Model file for the job. Use its own axes, mm. Round coordinates to 2 decimals unless told otherwise and drop trailing zeros. Loops run counter-clockwise (first coordinate to the right, second up) from the corner with the lowest first, then second, coordinate; pieces in that order, holes last. Notation, with made-up numbers: (38.25, 41.5) -> (92.25, 41.5) arc R20 cw to (92.25, 64.5) -> close; hole circle Ø10 at (5, 58). An arc over 180 degrees is marked (long way). Use a Markdown table: item, result.
from build123d import *

# Parameters (mm, degrees)
BOSS_EXTRUDE3_DEPTH = 200
CHAMFER2_SIZE       = 18
CHAMFER3_SIZE       = 18
SKETCH6_W           = 200
SKETCH6_H           = 8
CUT_EXTRUDE2_DEPTH  = 4
SKETCH7_W           = 200
SKETCH7_H           = 8
CUT_EXTRUDE3_DEPTH  = 4
SKETCH8_R           = 1.4
CUT_EXTRUDE4_DEPTH  = 3
SKETCH9_R           = 2.1
CUT_EXTRUDE5_DEPTH  = 6
SKETCH10_R          = 2.1
CUT_EXTRUDE6_DEPTH  = 6
CUT_EXTRUDE7_DEPTH  = 4
SKETCH12_W          = 4
SKETCH12_H          = 10
SKETCH12_W_2        = 10
SKETCH12_H_2        = 4
CUT_EXTRUDE8_DEPTH  = 14
FILLET1_R           = 4
FILLET2_R           = 4
SKETCH13_W          = 4
SKETCH13_H          = 10
SKETCH13_W_2        = 10
SKETCH13_H_2        = 4
CUT_EXTRUDE9_DEPTH  = 14
FILLET3_R           = 4
SKETCH14_R          = 2.1
CUT_EXTRUDE10_DEPTH = 4
SKETCH15_R          = 2.1
CUT_EXTRUDE11_DEPTH = 4
SKETCH16_R          = 2.1
CUT_EXTRUDE12_DEPTH = 4


with BuildPart() as part:
    # Sketch5 → Boss-Extrude3 (new body)
    with BuildSketch(Plane(origin=(0, 0, 0), x_dir=(0, 0, -1), z_dir=(1, 0, 0))):
        Polygon((0, 0), (0, 36), (8, 36), (8, 8), (36, 8), (36, 0), align=None)
    extrude(amount=BOSS_EXTRUDE3_DEPTH)

    # Chamfer2
    chamfer2_edges = [part.edges().sort_by_distance(p)[0] for p in [
        (100, 8, -8),
    ]]
    chamfer(chamfer2_edges, length=CHAMFER2_SIZE)

    # Chamfer3
    chamfer3_edges = [part.edges().sort_by_distance(p)[0] for p in [
        (100, 0, 0),
    ]]
    chamfer(chamfer3_edges, length=CHAMFER3_SIZE)

    # Sketch6 → Cut-Extrude2 (cut)
    with BuildSketch(Plane(origin=(0, 0, 0), x_dir=(-1, 0, 0), z_dir=(0, -1, 0))):
        with Locations((-100, 32)):
            Rectangle(SKETCH6_W, SKETCH6_H)
    extrude(amount=-CUT_EXTRUDE2_DEPTH, mode=Mode.SUBTRACT)

    # Sketch7 → Cut-Extrude3 (cut)
    with BuildSketch(Plane.XY):
        with Locations((100, 32)):
            Rectangle(SKETCH7_W, SKETCH7_H)
    extrude(amount=-CUT_EXTRUDE3_DEPTH, mode=Mode.SUBTRACT)

    # Sketch8 → Cut-Extrude4 (cut)
    with BuildSketch(Plane(origin=(0, 17, -17), x_dir=(-1, 0, 0), z_dir=(0, 0.7071067811865438, -0.7071067811865512))):
        with Locations(Location((-182.5, 0, 0), (0, 0, 90))):
            Circle(SKETCH8_R)
        with Locations(Location((-167.5, 0, 0), (0, 0, 90))):
            Circle(SKETCH8_R)
        with Locations(Location((-152.5, 0, 0), (0, 0, 90))):
            Circle(SKETCH8_R)
        with Locations(Location((-137.5, 0, 0), (0, 0, 90))):
            Circle(SKETCH8_R)
        with Locations(Location((-122.5, 0, 0), (0, 0, 90))):
            Circle(SKETCH8_R)
        with Locations(Location((-107.5, 0, 0), (0, 0, 90))):
            Circle(SKETCH8_R)
        with Locations(Location((-92.5, 0, 0), (0, 0, 90))):
            Circle(SKETCH8_R)
        with Locations(Location((-77.5, 0, 0), (0, 0, 90))):
            Circle(SKETCH8_R)
        with Locations(Location((-62.5, 0, 0), (0, 0, 90))):
            Circle(SKETCH8_R)
        with Locations(Location((-47.5, 0, 0), (0, 0, 90))):
            Circle(SKETCH8_R)
        with Locations(Location((-32.5, 0, 0), (0, 0, 90))):
            Circle(SKETCH8_R)
        with Locations(Location((-17.5, 0, 0), (0, 0, 90))):
            Circle(SKETCH8_R)
    extrude(amount=-CUT_EXTRUDE4_DEPTH, mode=Mode.SUBTRACT)

    # Sketch9 → Cut-Extrude5 (cut)
    with BuildSketch(Plane(origin=(0, 17, -17), x_dir=(-1, 0, 0), z_dir=(0, 0.7071067811865438, -0.7071067811865512))):
        with Locations(Location((-73, -10, 0), (0, 0, 90))):
            Circle(SKETCH9_R)
        with Locations(Location((-127, -10, 0), (0, 0, 90))):
            Circle(SKETCH9_R)
        with Locations(Location((-127, 10, 0), (0, 0, 90))):
            Circle(SKETCH9_R)
        with Locations(Location((-73, 10, 0), (0, 0, 90))):
            Circle(SKETCH9_R)
    extrude(amount=-CUT_EXTRUDE5_DEPTH, mode=Mode.SUBTRACT)

    # Sketch10 → Cut-Extrude6 (cut)
    with BuildSketch(Plane(origin=(0, 17, -17), x_dir=(-1, 0, 0), z_dir=(0, 0.7071067811865438, -0.7071067811865512))):
        with Locations(Location((-89, -10, 0), (0, 0, 90))):
            Circle(SKETCH10_R)
        with Locations(Location((-111, -10, 0), (0, 0, 90))):
            Circle(SKETCH10_R)
        with Locations(Location((-111, 10, 0), (0, 0, 90))):
            Circle(SKETCH10_R)
        with Locations(Location((-89, 10, 0), (0, 0, 90))):
            Circle(SKETCH10_R)
    extrude(amount=-CUT_EXTRUDE6_DEPTH, mode=Mode.SUBTRACT)

    # Sketch11 → Cut-Extrude7 (cut)
    with BuildSketch(Plane(origin=(0, 17, -17), x_dir=(-1, 0, 0), z_dir=(0, 0.7071067811865438, -0.7071067811865512))):
        Polygon((0, -12), (-14, 0), (0, 12), align=None)
        Polygon((-200, 12), (-186, 0), (-200, -12), align=None)
    extrude(amount=-CUT_EXTRUDE7_DEPTH, mode=Mode.SUBTRACT)

    # Sketch12 → Cut-Extrude8 (cut)
    with BuildSketch(Plane(origin=(200, 0, 0), x_dir=(0, 0, -1), z_dir=(1, 0, 0))):
        with Locations((2, 23)):
            Rectangle(SKETCH12_W, SKETCH12_H)
        with Locations((23, 2)):
            Rectangle(SKETCH12_W_2, SKETCH12_H_2)
    extrude(amount=-CUT_EXTRUDE8_DEPTH, mode=Mode.SUBTRACT)

    # Fillet1
    fillet1_edges = [part.edges().sort_by_distance(p)[0] for p in [
        (14, 15.585786438, -15.585786438),
        (186, 15.585786438, -15.585786438),
    ]]
    fillet(fillet1_edges, radius=FILLET1_R)

    # Fillet2
    fillet2_edges = [part.edges().sort_by_distance(p)[0] for p in [
        (186, 18, -2),
        (186, 2, -18),
    ]]
    fillet(fillet2_edges, radius=FILLET2_R)

    # Sketch13 → Cut-Extrude9 (cut)
    with BuildSketch(Plane.ZY):
        with Locations((-2, 23)):
            Rectangle(SKETCH13_W, SKETCH13_H)
        with Locations((-23, 2)):
            Rectangle(SKETCH13_W_2, SKETCH13_H_2)
    extrude(amount=-CUT_EXTRUDE9_DEPTH, mode=Mode.SUBTRACT)

    # Fillet3
    fillet3_edges = [part.edges().sort_by_distance(p)[0] for p in [
        (14, 18, -2),
        (14, 2, -18),
    ]]
    fillet(fillet3_edges, radius=FILLET3_R)

    # Sketch14 → Cut-Extrude10 (cut)
    with BuildSketch(Plane.XY.offset(-4)):
        with Locations((192, 24)):
            Circle(SKETCH14_R)
        with Locations((8, 24)):
            Circle(SKETCH14_R)
    extrude(amount=-CUT_EXTRUDE10_DEPTH, mode=Mode.SUBTRACT)

    # Sketch15 → Cut-Extrude11 (cut)
    with BuildSketch(Plane(origin=(0, 4, 0), x_dir=(-1, 0, 0), z_dir=(0, -1, 0))):
        with Locations(Location((-8, 24, 0), (0, 0, 90))):
            Circle(SKETCH15_R)
        with Locations(Location((-192, 24, 0), (0, 0, 90))):
            Circle(SKETCH15_R)
    extrude(amount=-CUT_EXTRUDE11_DEPTH, mode=Mode.SUBTRACT)

    # Sketch16 → Cut-Extrude12 (cut)
    with BuildSketch(Plane(origin=(0, 14.171572875, -14.171572875), x_dir=(-1, 0, 0), z_dir=(0, 0.7071067811865438, -0.7071067811865513))):
        with Locations(Location((-6, 0, 0), (0, 0, 90))):
            Circle(SKETCH16_R)
        with Locations(Location((-194, 0, 0), (0, 0, 90))):
            Circle(SKETCH16_R)
    extrude(amount=-CUT_EXTRUDE12_DEPTH, mode=Mode.SUBTRACT)


solid = part.part
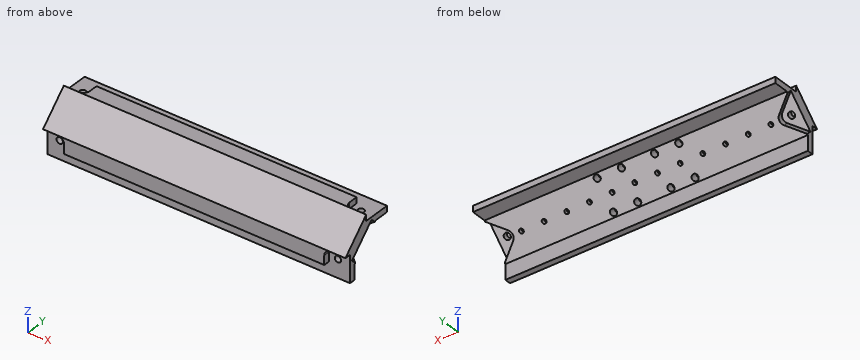
Q1. Drill centre lines: L1, parallel to X at y = 24, z = -6.4; L2, parallel to Z at x = 192, y = 6; L3, parallel to X at y = 22.5, z = -9. Where is each one in solid material? Low to high. Write a range as from..to.
Results list:
| item | result |
|---|---|
| L1 | x = 0..5.9, 10.1..189.9, 194.1..200 |
| L2 | z = -36..-26.1, -21.9..-12 |
| L3 | x = 2.86..70.95, 75.05..86.95, 91.05..108.95, 113.05..124.95, 129.05..197.14 |
Q2. Band-saw the part on B-B, the plane y = 30. Give the cut face in (x, z).
Results list:
| item | result |
|---|---|
| outline | (0, -8) -> (200, -8) -> (200, -4) -> (0, -4) -> close |
Q3. Flat gauge pins, fed straight in: pin 1 (4 mm diameter, centred on x = 63, z = -9, fed in from -Y); pin 2 (2.5 mm diameter, centred on x = 192, z = -24, fed in from -Y); pin 3 (1.2 mm diameter, centred on x = 8.5, y = 24, fed in from +Z); pin 4 (6 mm diameter, centred on y = 18, z = -22.5, fed in from -X). Where does each tip first touch, or does it go through?
Results list:
| item | result |
|---|---|
| pin 1 | stops at y = 7 |
| pin 2 | stops at y = 8 |
| pin 3 | stops at z = -8 |
| pin 4 | passes through |
Q4. Band-saw the part on A-A, the plane x = 134. Give the cut face in (y, z), plus the area to 3 significant figures.
Results list:
| item | result |
|---|---|
| outline | (0, -28) -> (4, -28) -> (4, -36) -> (8, -36) -> (8, -26) -> (26, -8) -> (36, -8) -> (36, -4) -> (28, -4) -> (28, 0) -> (18, 0) -> (0, -18) -> close |
| area | 448 mm² |
Q5. Band-saw the part on C-C, the plane z = -33.5. Give the cut face in (x, y).
Results list:
| item | result |
|---|---|
| outline | (0, 4) -> (200, 4) -> (200, 8) -> (0, 8) -> close |
